```python
from build123d import *

# Parameters (mm, degrees)
F0_R            = 60.8062922789
F1_DEPTH        = 15.24
F3_DEPTH        = 15.241
F3_COPIES_COUNT = 20


# Not quite as in the source:
# - a pattern or mirror of a feature is missing from the dataset's text; its kind, count and spacing are read off the source's solid


with BuildPart() as f1:
    # F0 (on Front) → F1 (new body)
    with BuildSketch(Plane.XZ):
        Circle(F0_R)
    extrude(amount=F1_DEPTH)

    # F2 (on face) → F3 (cut, through all)
    with BuildSketch(Plane.XZ.offset(15.24)):
        with BuildLine():
            ThreePointArc((-10.0692585111, 64.2209947109), (-8.0132671596, 62.5211963323), (-6.2964195687, 60.4794203124))
            ThreePointArc((-6.2964195687, 60.4794203124), (0, 60.8062922789), (6.2964195687, 60.4794203124))
            ThreePointArc((6.2964195687, 60.4794203124), (8.0132671596, 62.5211963323), (10.0692585111, 64.2209947109))
            Line((10.0692585111, 64.2209947109), (-10.0692585111, 64.2209947109))
        make_face()
        with BuildLine():
            ThreePointArc((-6.2964195687, 60.4794203124), (-4.802623185, 57.7701032506), (-3.9057508111, 54.8091158271))
            Line((-3.9057508111, 54.8091158271), (0, 54.8091158271))
            Line((0, 54.8091158271), (3.9057508111, 54.8091158271))
            ThreePointArc((3.9057508111, 54.8091158271), (4.802623185, 57.7701032506), (6.2964195687, 60.4794203124))
            ThreePointArc((6.2964195687, 60.4794203124), (0, 60.8062922789), (-6.2964195687, 60.4794203124))
        make_face()
    f3 = extrude(amount=-F3_DEPTH, mode=Mode.SUBTRACT)

    # F3_copies: F3 ×20 about axis
    f3_copies_axis = Axis((0, 0, 0), (0, 1, 0))
    for i in range(1, F3_COPIES_COUNT):
        add(f3.rotate(f3_copies_axis, i * 360 / F3_COPIES_COUNT), mode=Mode.SUBTRACT)


solid = f1.part
```
Can you work these out from the model? Positions are in its coordinate system, mm. A direction names the side the tool comes from. Coordinates: 2 decimals unless noted, no trailing zeros. Loops run counter-clockwise (first coordinate to the right, second up) from the corner with the lowest first, then second, coordinate; pieces in that order, holes last.
Item 1: Suppose I cut it at A-A (z = 2). Please give me the cut outline in (x, y).
Answers below:
outline: (-54.81, -15.24) - (54.81, -15.24) - (54.81, 0) - (-54.81, 0) - close
Item 2: Suppose I cut it at B-B (x = 18.5). Please give me the cut outline in (y, z), then the cut area to 3 significant figures.
Answers below:
outline: (-15.24, -51.62) - (0, -51.62) - (0, 51.62) - (-15.24, 51.62) - close
area: 1,570 mm2
Item 3: Which directions (+Z, -Z, +X, -X, +Y, -Y) give clear straight access to the entire face, cutting with the end or side of a thin tool? Please do faces 1 (the face through (44.31, -7.73, 32.26)), 2 (the face through (-30.06, -7.73, 49.52)), 3 (the face through (-49.6, -7.73, 30.08)), 4 (the face through (-4.786, -7.727, -57.73)).
Answers below:
face 1: +Y, -Y
face 2: -X, +Y, -Y
face 3: +Z, +Y, -Y
face 4: -Z, +Y, -Y
Item 4: If we mould it in two halves opening along Z, with no side actions, what happens to faces 5 (the face through (49.52, -7.73, 30.06)), 6 (the face through (-9.56, -7.51, -60.05)), 7 (the face through (-53.491, -7.727, -22.448))? For each: released by +Z, released by -Z, zero draft, split by the parting line, or undercut.
Answers below:
face 5: released by +Z
face 6: released by -Z
face 7: undercut
Item 5: I'm going to push flat-ended pins straight in: pin 1 (8 mm diameter, centred on y = -11, z = -42, fed in from +X); pin 2 (3 mm diameter, centred on x = -12.5, y = -4.5, fed in from -Z); pin 3 (2.5 mm diameter, centred on y = -6, z = 0.5, fed in from +X); pin 4 (4 mm diameter, centred on x = -33.5, z = -47, fed in from +Y). Where does each tip first touch, or does it pass through?
Answers below:
pin 1: stops at x = 45.23
pin 2: stops at z = -59.8
pin 3: stops at x = 54.81
pin 4: passes through
Item 6: Please list where these lines run through material, in increasing order: L1, parallel to X at y = -4, z = 42.5; L2, parallel to X at y = -8, z = 3.
Answers below:
L1: x = -43.49 to -35.88, -34.75 to 34.75, 35.88 to 43.49
L2: x = -54.81 to 54.81
